Source: CAD feature listing. Evaluate the final solid. Frame: model axes, mm. A direction names the side the tool comes from. Round coordinates to 2 decimals unless told otherwise and drop trailing zeros. Write each loop counter-clockwise with the first axis right and the second up, starting at its lowest first coordinate (ties: lowest second). Pieces come first, ordered by that corner, then holes. Notation, with made-up numbers: (57.25, -35) - (109.25, -35) arc R12 cw to (109.25, -18) - close; hole circle Ø3 at (41, 49.25). An arc over 180 degrees is marked (long way). Write item = value, one per line. Start each with the question number.
Autodesk Fusion 360 part; units mm, degrees
sketch "Sketch1" plane through (0, 0, 0) normal (0, 0, 1) x (1, 0, 0)
  line L0 (-75, 55) -> (65.2, 55)
  line L1 (65.2, 55) -> (65.2, -55.2)
  line L2 (65.2, -55.2) -> (-75, -55.2)
  line L3 (-75, -55.2) -> (-75, 55)
  dimension "d1" = 140.2
  dimension "d2" = 110.2
extrude "Extrude1" add sketch "Sketch1" along normal blind 5
sketch "Sketch2" plane through (0, 0, 0) normal (0, 0, -1) x (1, 0, 0)
  line L0 (65.2, 55.2) -> (-75, 55.2)
  line L1 (-75, 55.2) -> (-75, -55)
  line L2 (-75, -55) -> (65.2, -55)
  line L3 (65.2, -55) -> (65.2, 55.2)
  line L4 (65.2, -55) -> (45, -55)
  line L5 (45, -55) -> (45, -34.8)
  line L6 (45, -34.8) -> (65.2, -34.8)
  line L7 (65.2, -34.8) -> (65.2, -55)
  line L8 (-75, -55) -> (-54.8, -55)
  line L9 (-54.8, -55) -> (-54.8, -34.8)
  line L10 (-54.8, -34.8) -> (-75, -34.8)
  line L11 (-75, -34.8) -> (-75, -55)
  line L12 (5.2, -55) -> (-15, -55)
  line L13 (-15, -55) -> (-15, -34.8)
  line L14 (-15, -34.8) -> (5.2, -34.8)
  line L15 (5.2, -34.8) -> (5.2, -55)
  line L16 (65.2, 55.2) -> (45, 55.2)
  line L17 (45, 55.2) -> (45, 35)
  line L18 (45, 35) -> (65.2, 35)
  line L19 (65.2, 35) -> (65.2, 55.2)
  line L20 (5.2, 55.2) -> (-15, 55.2)
  line L21 (-15, 55.2) -> (-15, 35)
  line L22 (-15, 35) -> (5.2, 35)
  line L23 (5.2, 35) -> (5.2, 55.2)
  line L24 (-75, 55.2) -> (-54.8, 55.2)
  line L25 (-54.8, 55.2) -> (-54.8, 35)
  line L26 (-54.8, 35) -> (-75, 35)
  line L27 (-75, 35) -> (-75, 55.2)
  line L28 (60.2, -50) -> (50, -50)
  line L29 (50, -50) -> (50, -39.8)
  line L30 (50, -39.8) -> (60.2, -39.8)
  line L31 (60.2, -39.8) -> (60.2, -50)
  line L32 (0.2, -50) -> (-10, -50)
  line L33 (-10, -50) -> (-10, -39.8)
  line L34 (-10, -39.8) -> (0.2, -39.8)
  line L35 (0.2, -39.8) -> (0.2, -50)
  line L36 (-59.8, -50) -> (-70, -50)
  line L37 (-70, -50) -> (-70, -39.8)
  line L38 (-70, -39.8) -> (-59.8, -39.8)
  line L39 (-59.8, -39.8) -> (-59.8, -50)
  line L40 (60.2, 40) -> (50, 40)
  line L41 (50, 40) -> (50, 50.2)
  line L42 (50, 50.2) -> (60.2, 50.2)
  line L43 (60.2, 50.2) -> (60.2, 40)
  line L44 (0.2, 40) -> (-10, 40)
  line L45 (-10, 40) -> (-10, 50.2)
  line L46 (-10, 50.2) -> (0.2, 50.2)
  line L47 (0.2, 50.2) -> (0.2, 40)
  line L48 (-59.8, 40) -> (-70, 40)
  line L49 (-70, 40) -> (-70, 50.2)
  line L50 (-70, 50.2) -> (-59.8, 50.2)
  line L51 (-59.8, 50.2) -> (-59.8, 40)
  dimension "d5" = 20.2
  dimension "d6" = 20.2
  dimension "d7" = 20.2
  dimension "d8" = 39.8
  dimension "d9" = 20.2
  dimension "d10" = 20.2
  dimension "d11" = 39.8
  dimension "d12" = 20.2
  dimension "d13" = 20.2
  dimension "d14" = 20.2
  dimension "d15" = 20.2
  dimension "d16" = 39.8
  dimension "d17" = 20.2
  dimension "d18" = 39.8
  dimension "d19" = 20.2
  dimension "d20" = 20.2
  dimension "d21" = 5
  dimension "d22" = 5
  dimension "d23" = 5
  dimension "d24" = 5
  dimension "d25" = 5
  dimension "d26" = 5
  dimension "d27" = 5
  dimension "d28" = 5
  dimension "d29" = 5
  dimension "d30" = 5
  dimension "d31" = 5
  dimension "d32" = 5
  dimension "d33" = 5
  dimension "d34" = 5
  dimension "d35" = 5
  dimension "d36" = 5
  dimension "d37" = 5
  dimension "d38" = 5
  dimension "d39" = 5
  dimension "d40" = 5
  dimension "d41" = 5
  dimension "d42" = 5
  dimension "d43" = 5
  dimension "d44" = 5
extrude "Extrude2" cut sketch "Sketch2" against normal blind 2.5 contours L28 L29 L30 L31 | L32 L33 L34 L35 | L36 L37 L38 L39 | L40 L41 L42 L43 | L44 L45 L46 L47 | L48 L49 L50 L51
extrude "Extrude3" add sketch "Sketch2" along normal blind 10 contours L0 L3 L16 L17 L18 L19 | L0 L20 L21 L22 L23 | L2 L3 L4 L5 L6 L7 | L0 L1 L24 L25 L26 L27 | L2 L12 L13 L14 L15 | L1 L2 L8 L9 L10 L11
sketch "Sketch3" plane through (0, 0, 5) normal (0, 0, 1) x (-1, 0, 0)
  line L0 (75, 55.2) -> (-65.2, 55.2)
  line L1 (-65.2, 55.2) -> (-65.2, -55)
  line L2 (-65.2, -55) -> (75, -55)
  line L3 (75, -55) -> (75, 55.2)
  line L4 (14.9, -19.9) -> (-5.1, -19.9)
  line L5 (-5.1, -19.9) -> (-5.1, 20.1)
  line L6 (-5.1, 20.1) -> (14.9, 20.1)
  line L7 (14.9, 20.1) -> (14.9, -19.9)
  dimension "d49" = 20
  dimension "d50" = 40
  dimension "d51" = 110.2
  dimension "d52" = 140.2
  dimension "d53" = 35.1
  dimension "d54" = 35.1
  dimension "d55" = 60.1
  dimension "d56" = 60.1
extrude "Extrude4" add sketch "Sketch3" along normal blind 5 contours L4 L5 L6 L7
fillet "Fillet1" radius 2 4 edges at (-75, -55.2, -2.5) (65.2, -55.2, -2.5) (65.2, 55, -2.5) (-75, 55, -2.5)
fillet "Fillet2" radius 2 4 edges at (5.1, -20.1, 7.5) (-14.9, -20.1, 7.5) (5.1, 19.9, 7.5) (-14.9, 19.9, 7.5)
(1) Section B-B (z = -5.5). Count the separate pieces of the cut face and the enclosed holes in it, plus the area to 3 significant figures.
(2) Section D-D (x = 41). Return the cut outline in (y, z), plus the area to 3 significant figures.
(3) Pull-direction query (X, two-part tool) for faces 1 (the flat face through (55, 45, 2.5)), 2 (the flat face through (65.2, 1, 1)), 3 (the flat face through (-65, -52, -10)); classes: +X half, -X half, draft (parallel to the pull), parting line (faces both ways), or undercut.
(4) Section C-C (z = 7.25). Return the cut outline in (x, y), plus the area to 3 significant figures.
(5) Contact query for flat-ended pins moving along their axis: P1, Ø1.5, axis at y = 5, z = 6.5, coming from the +X side; P2, Ø6, axis at x = 11, y = -31.5, coming from the -Z side; P3, Ø5, axis at x = -5.5, y = -46.5, coming from the -Z side. Output: stop coordinate, or through.
(6) Section A-A (y = -12.5). Return the cut outline in (x, z).
(7) Ray query, L1, parallel to X at y = -45, z = -5.75; L2, parallel to Y at x = 56, z = 1.25; L3, parallel to Y at x = 51, z = -2.5. Return the intervals inside material, ascending. Write a range as from..to.
(8) Reachability of faces 4 (the flat face through (-5, 19.9, 7)), 5 (the flat face through (45, 45, -5)), 6 (the flat face through (55, -52, -10)), 7 (the flat face through (-65, -45, 2.5)), 8 (the flat face through (-65, -35, -5)) from +Z, -Z, +X, -X, +Y, -Y: full face, straight path, thin tool, end or side. Return the list, or none.
Solution:
q1.separate_pieces = 6
q1.enclosed_holes = 6
q1.area = 1,820 mm^2
q2.outline = (-55.2, 0) - (55, 0) - (55, 5) - (-55.2, 5) - close
q2.area = 551 mm^2
q3.face_1 = undercut
q3.face_2 = +X half
q3.face_3 = draft
q4.outline = (-14.9, -18.1) arc R2 ccw to (-12.9, -20.1) - (3.1, -20.1) arc R2 ccw to (5.1, -18.1) - (5.1, 17.9) arc R2 ccw to (3.1, 19.9) - (-12.9, 19.9) arc R2 ccw to (-14.9, 17.9) - close
q4.area = 797 mm^2
q5.P1 = 5.1
q5.P2 = 0
q5.P3 = 2.5
q6.outline = (-75, 0) - (65.2, 0) - (65.2, 5) - (5.1, 5) - (5.1, 10) - (-14.9, 10) - (-14.9, 5) - (-75, 5) - close
q7.L1 = -75..-70, -59.8..-54.8, -15..-10, 0.2..5.2, 45..50, 60.2..65.2
q7.L2 = -55.2..-50.2, -40..39.8, 50..55
q7.L3 = -55.2..-50.2, -40..-35, 34.8..39.8, 50..55
q8.face_4 = +Z, +X, -X, +Y
q8.face_5 = -Z, +Y, -Y
q8.face_6 = -Z, +X, -X, +Y, -Y
q8.face_7 = -Z
q8.face_8 = -Z, +X, -X
